Verification items for the finished model (mm, model axes). Face numbers are marked on the shaded views. A direction names the side the tool comes from. Round coordinates to 2 decimals unless told otherwise and drop trailing zeros. Order: outer loops, then holes, each group sorted by start corner. A loop starts at its lowest first (then second) coordinate and runs counter-clockwise, first axis right, second up. Notation, with made-up numbers: M 50.5,59 L 80.5,59 A34 ccw 80.5,89 Z; hole C 32.5,4.25 d2. An arc over 180 degrees is marked long. Write item = value, one per line. Start each with the question number.
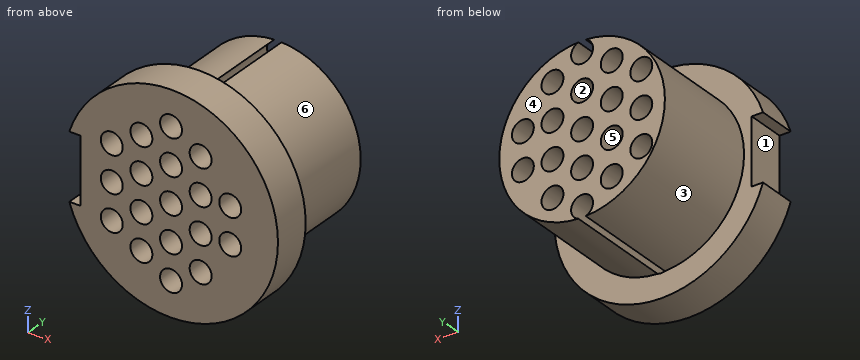
Autodesk Inventor part; units mm, degrees
ref_plane "YZ Plane" through (0, 0, 0) normal (1, 0, 0) x (0, 1, 0)
ref_plane "XZ Plane" through (0, 0, 0) normal (0, 1, 0) x (-1, 0, 0)
ref_plane "XY Plane" through (0, 0, 0) normal (0, 0, 1) x (1, 0, 0)
sketch "Sketch1" plane through (0, 0, 0) normal (0, 1, 0) x (-1, 0, 0)
  point P0 (0, 0)
sketch "Sketch2" plane through (0, 0, 0) normal (0, 1, 0) x (-1, 0, 0)
  line L0 (0, -0.6) -> (0, -2.7)
  line L1 (0, -2.7) -> (0, -3.3)
  line L2 (0, -3.9) -> (0, -6)
  line L3 (0, -6) -> (0, -6.6)
  line L4 (0, 0.6) -> (0, 3.3)
  line L5 (0, 3.9) -> (0, 6.6)
  line L6 (0, -0.6) -> (0, -1.65)
  line L7 (0, -0.6) -> (0, -1.65)
  line L8 (0, -1.65) -> (2.7, -1.65)
  line L9 (2.7, -1.65) -> (2.7, -3.75)
  line L10 (2.7, -3.75) -> (2.7, -4.95)
  line L11 (2.7, -1.05) -> (2.7, 1.05)
  line L12 (2.7, 1.05) -> (2.7, 1.65)
  line L13 (2.7, 2.25) -> (2.7, 4.95)
  line L14 (2.7, 0) -> (5.4, 0)
  line L15 (5.4, 0) -> (5.4, -3.3)
  line L16 (5.4, 0) -> (5.4, 3.3)
  line L17 (0, -1.65) -> (-2.7, -1.65)
  line L18 (-2.7, -1.65) -> (-2.7, -4.35)
  line L19 (-2.7, -4.35) -> (-2.7, -4.95)
  line L20 (-2.7, -1.65) -> (-2.7, 1.65)
  line L21 (-2.7, 1.65) -> (-2.7, 4.95)
  line L22 (-2.7, -1.65) -> (-5.4, -1.65)
  line L23 (-2.7, 1.65) -> (-5.4, 1.65)
  circle A0 centre (0, -6.6) radius 1
  circle A1 centre (2.7, -4.95) radius 1
  circle A2 centre (-2.7, -4.95) radius 1
  circle A3 centre (0, -3.3) radius 1
  circle A4 centre (5.4, -3.3) radius 1
  circle A5 centre (2.7, -1.65) radius 1
  circle A6 centre (-2.7, -1.65) radius 1
  circle A7 centre (-5.4, -1.65) radius 1
  circle A8 centre (0, 0) radius 1
  circle A9 centre (5.4, 0) radius 1
  circle A10 centre (2.7, 1.65) radius 1
  circle A11 centre (5.4, 3.3) radius 1
  circle A12 centre (0, 3.3) radius 1
  circle A13 centre (-2.7, 1.65) radius 1
  circle A14 centre (-5.4, 1.65) radius 1
  circle A15 centre (-2.7, 4.95) radius 1
  circle A16 centre (2.7, 4.95) radius 1
  circle A17 centre (0, 6.6) radius 1
  circle A18 centre (0, 0) radius 9.75
  line L24 (9.75, 0) -> (8.25, 0)
  line L25 (8.25, 0) -> (8.25, 3)
  line L26 (8.25, 3) -> (10.1008, 3)
  line L27 (8.25, 0) -> (8.25, -3)
  line L28 (8.25, -3) -> (10.4334, -3)
  point P0 (-2, 10.0571)
  point P1 (2, 10.0571)
  point P2 (9.277, 3)
  point P3 (9.277, -3)
  dimension "d127" = 19.5
  dimension "d53" = 2.1
  dimension "d54" = 0.6
  dimension "d56" = 2.1
  dimension "d57" = 0.6
  dimension "d59" = 2.7
  dimension "d61" = 2.7
  dimension "d63" = 1.05
  dimension "d64" = 2.7
  dimension "d66" = 2.1
  dimension "d67" = 1.2
  dimension "d69" = 2.1
  dimension "d70" = 0.6
  dimension "d72" = 2.7
  dimension "d74" = 2.7
  dimension "d78" = 2.7
  dimension "d80" = 2.7
  dimension "d81" = 0.6
  dimension "d85" = 2.7
  dimension "d87" = 2.7
  dimension "d91" = 2
  dimension "d92" = 2
  dimension "d93" = 2
  dimension "d94" = 2
  dimension "d95" = 2
  dimension "d96" = 2
  dimension "d97" = 2
  dimension "d98" = 2
  dimension "d99" = 2
  dimension "d100" = 2
  dimension "d101" = 2
  dimension "d102" = 2
  dimension "d103" = 2
  dimension "d104" = 2
  dimension "d105" = 2
  dimension "d106" = 2
  dimension "d107" = 2
  dimension "d108" = 2
  dimension "d128" = 1.5
  dimension "d129" = 3
  dimension "d130" = 3
extrude "Extrusion1" add sketch "Sketch2" along normal blind 3.5 contours L26 L25 L27 L28 A18
sketch "Sketch3" plane through (0, 3.5, 0) normal (0, 1, 0) x (-1, 0, 0)
  circle A0 centre (0, 0) radius 7.55
  line L0 (0, -0.6) -> (0, -2.7)
  line L1 (0, -2.7) -> (0, -3.3)
  line L2 (0, -3.9) -> (0, -6)
  line L3 (0, -6) -> (0, -6.6)
  line L4 (0, 0.6) -> (0, 3.3)
  line L5 (0, 3.9) -> (0, 6.6)
  line L6 (0, -0.6) -> (0, -1.65)
  line L7 (0, -0.6) -> (0, -1.65)
  line L8 (0, -1.65) -> (2.7, -1.65)
  line L9 (2.7, -1.65) -> (2.7, -3.75)
  line L10 (2.7, -3.75) -> (2.7, -4.95)
  line L11 (2.7, -1.05) -> (2.7, 1.05)
  line L12 (2.7, 1.05) -> (2.7, 1.65)
  line L13 (2.7, 2.25) -> (2.7, 4.95)
  line L14 (2.7, 0) -> (5.4, 0)
  line L15 (5.4, 0) -> (5.4, -3.3)
  line L16 (5.4, 0) -> (5.4, 3.3)
  line L17 (0, -1.65) -> (-2.7, -1.65)
  line L18 (-2.7, -1.65) -> (-2.7, -4.35)
  line L19 (-2.7, -4.35) -> (-2.7, -4.95)
  line L20 (-2.7, -1.65) -> (-2.7, 1.65)
  line L21 (-2.7, 1.65) -> (-2.7, 4.95)
  line L22 (-2.7, -1.65) -> (-5.4, -1.65)
  line L23 (-2.7, 1.65) -> (-5.4, 1.65)
  circle A1 centre (0, -6.6) radius 1
  circle A2 centre (-2.7, -4.95) radius 1
  circle A3 centre (0, -3.3) radius 1
  circle A4 centre (2.7, -4.95) radius 1
  circle A5 centre (5.4, -3.3) radius 1
  circle A6 centre (2.7, -1.65) radius 1
  circle A7 centre (-2.7, -1.65) radius 1
  circle A8 centre (-5.4, -1.65) radius 1
  circle A9 centre (5.4, 0) radius 1
  circle A10 centre (0, 0) radius 1
  circle A11 centre (2.7, 1.65) radius 1
  circle A12 centre (-2.7, 1.65) radius 1
  circle A13 centre (-5.4, 1.65) radius 1
  circle A14 centre (0, 3.3) radius 1
  circle A15 centre (5.4, 3.3) radius 1
  circle A16 centre (2.7, 4.95) radius 1
  circle A17 centre (-2.7, 4.95) radius 1
  circle A18 centre (0, 6.6) radius 1
  point P0 (-0.3339, 7.5426)
  point P1 (-0.3339, -7.5426)
  point P2 (0.3339, -7.5426)
  point P3 (0.3339, 7.5426)
  dimension "d12" = 2.1
  dimension "d13" = 0.6
  dimension "d15" = 2.1
  dimension "d16" = 0.6
  dimension "d18" = 2.7
  dimension "d20" = 2.7
  dimension "d22" = 1.05
  dimension "d23" = 2.7
  dimension "d25" = 2.1
  dimension "d26" = 1.2
  dimension "d28" = 2.1
  dimension "d29" = 0.6
  dimension "d31" = 2.7
  dimension "d33" = 2.7
  dimension "d37" = 2.7
  dimension "d39" = 2.7
  dimension "d40" = 0.6
  dimension "d44" = 2.7
  dimension "d46" = 2.7
  dimension "d109" = 2
  dimension "d110" = 2
  dimension "d111" = 2
  dimension "d112" = 2
  dimension "d113" = 2
  dimension "d114" = 2
  dimension "d115" = 2
  dimension "d116" = 2
  dimension "d117" = 2
  dimension "d118" = 2
  dimension "d119" = 2
  dimension "d120" = 2
  dimension "d121" = 2
  dimension "d122" = 2
  dimension "d123" = 2
  dimension "d124" = 2
  dimension "d125" = 2
  dimension "d126" = 2
extrude "Extrusion2" add sketch "Sketch3" along normal blind 10 contours A0 A1 L2 A3 L0 A10 L4 A14 L5 A18 | A18 L5 A14 L4 A10 L0 A3 L2 A1 A0
properties part number "inner Part of Adaptor"
1) Gauge pin test, flat ends, axial feed: P1, Ø1.2, axis at x = 0, z = -3.3, coming from the -Y side; P2, Ø1.5, axis at x = -2.5, y = 11.5, coming from the +Z side; P3, Ø4, axis at y = 1.5, z = -0.5, coming from the -X side; P4, Ø6, axis at x = -3.5, y = 12, coming from the -Z side. Record the tip position at first contact, or that the pin passes through.
2) Cross-section at A-A, the plane z = 0. Enter the section's corners in (x, y), then the cut area to 3 significant figures.
3) Cross-section at B-B, the plane y = 7.5. Give the number of separate pieces and of enclosed holes in the cut face, then the cut area to 3 significant figures.
4) Access from +Z, -Z, +X, -X, +Y, -Y to the whole of each face (thin tool, end or side, straight path). Record for the marked faces 1, 2 and 3.
5) Cross-section at D-D, the plane x = 2.5. Enter the section's corners in (y, z), then the cut area to 3 significant figures.
6) Release check for a two-part mould opening along Z. For the marked faces 4, 5 and 6 record: pulls with the +Z half, pulls with the -Z half, needs draft (parallel to the pull), parting line crosses it, or undercut.
7) Cross-section at C-C, the plane x = 5.4. Enter the section's corners in (y, z).
8) Scan lines: probe 1 along Z at (x, y) = (0, 7.5); probe 2 along Z at (x, y) = (-5.4, 8); probe 3 along X at (y, z) = (2, 0.5). Record each from-to range of solid material in increasing order.
Geometry results:
q1.P1 = through
q1.P2 = 7.34
q1.P3 = -8.25
q1.P4 = -7.53
q2.outline = M -8.25,0 L -6.4,0 L -6.4,13.5 L -7.55,13.5 L -7.55,3.5 L -8.25,3.5 Z; M -4.4,0 L -1,0 L -1,13.5 L -4.4,13.5 Z; M 1,0 L 9.75,0 L 9.75,3.5 L 7.55,3.5 L 7.55,13.5 L 1,13.5 Z
q2.area = 160 mm^2
q3.separate_pieces = 1
q3.enclosed_holes = 16
q3.area = 123 mm^2
q4.face_1 = -X, +Y, -Y
q4.face_2 = +Y, -Y
q4.face_3 = -X, +Y
q5.outline = M 0,-9.42 L 3.5,-9.42 L 3.5,-7.12 L 13.5,-7.12 L 13.5,-5.93 L 0,-5.93 Z; M 0,-3.97 L 13.5,-3.97 L 13.5,-2.63 L 0,-2.63 Z; M 0,-0.67 L 13.5,-0.67 L 13.5,0.67 L 0,0.67 Z; M 0,2.63 L 13.5,2.63 L 13.5,3.97 L 0,3.97 Z; M 0,5.93 L 13.5,5.93 L 13.5,7.12 L 3.5,7.12 L 3.5,9.42 L 0,9.42 Z
q5.area = 103 mm^2
q6.face_4 = needs draft
q6.face_5 = undercut
q6.face_6 = parting line crosses it
q7.outline = M 0,-8.12 L 3.5,-8.12 L 3.5,-5.28 L 13.5,-5.28 L 13.5,-2.65 L 0,-2.65 Z; M 0,-0.65 L 13.5,-0.65 L 13.5,0.65 L 0,0.65 Z; M 0,2.65 L 13.5,2.65 L 13.5,5.28 L 3.5,5.28 L 3.5,8.12 L 0,8.12 Z
q8.probe_1 = -5.6 to -4.3, -2.3 to -1, 1 to 2.3, 4.3 to 5.6
q8.probe_2 = -5.28 to -4.3, -2.3 to -1, 1 to 2.3, 4.3 to 5.28
q8.probe_3 = -8.25 to -6.27, -4.53 to -0.87, 0.87 to 9.74
